The model under review builds one solid part; all positions refer to its coordinate system, in mm. A direction names the side the tool comes from. Round coordinates to 2 decimals unless told otherwise and drop trailing zeros. Answer as CSV lines item,"result". Start each with the question number.
from build123d import *

# Parameters (mm, degrees)
EXTRUDE_1_DEPTH = 15


with BuildPart() as part:
    # 放样1: read off the stored shape, not the designer's step
    # 放样1: loft between two sections, ruled curve by curve
    loft_1_from = [
        Edge.make_bspline([(157.289403045, 194.319437241, 200), (545.928277528, -120.259368848, 200), (231.349471438, -508.898243331, 200), (-157.289403045, -194.319437241, 200), (-545.928277528, 120.259368848, 200), (-231.349471438, 508.898243331, 200), (157.289403045, 194.319437241, 200)], [0, 0, 0, 0, 0.5, 0.5, 0.5, 1, 1, 1, 1], 3, [1, 0.333333333, 0.333333333, 1, 0.333333333, 0.333333333, 1]),
    ]
    loft_1_to = [
        Edge.make_bspline([(42.317097013, 26.631997679, 0), (95.581092372, -58.002196347, 0), (10.946898346, -111.266191705, 0), (-42.317097013, -26.631997679, 0), (-95.581092372, 58.002196347, 0), (-10.946898346, 111.266191705, 0), (42.317097013, 26.631997679, 0)], [0, 0, 0, 0, 0.5, 0.5, 0.5, 1, 1, 1, 1], 3, [1, 0.333333333, 0.333333333, 1, 0.333333333, 0.333333333, 1]),
    ]
    loft_1 = Solid(Shell([*[Face.make_surface_from_curves(loft_1_from[k], loft_1_to[k]) for k in range(1)], Face(Wire(loft_1_from)), Face(Wire(loft_1_to))]))
    add(loft_1)

    # 草图4 → 凸台-拉伸1 (add)
    with BuildSketch(Plane.XY.offset(200)):
        Polygon((0, 250), (-250, 250), (-250, -250), (250, -250), (250, 250), align=None)
    extrude(amount=EXTRUDE_1_DEPTH)


solid = part.part
Item 1: For pin 1 (12 mm diameter, centred on x = 110.5, y = 12, fed in from -Z); pin 2 (8 mm diameter, centred on y = -93.5, z = 191, fed in from +X); pin 3 (4 mm diameter, centred on x = -9.5, z = 127.5, fed in from -Y), all flat-tipped, find the tip position at first contact; note any pin that passes through.
Item 2: Wall thickness on probe 1 along Z at (x, y) = (223.5, -191.5); probe 2 along X at (y, z) = (125, 129.5); probe 3 along Z at (x, y) = (-40.5, -96): over which ranges is each line inside the solid? List them lowest first. Write a range as [from, to].
Item 3: Tool access review of faces 1 (the flat face through (-200, 190, 200)), 2 (the flat face through (189, 200, 200)), 3 (the flat face through (198, -198, 200)), 4 (the flat face through (-200, -189, 200)): name each direction out of +Z, -Z, +X, -X, +Y, -Y from which nothing blocks a thin tool from reaching the whole face with its end or side.
Reported:
1,pin 1,"stops at z = 56.43"
1,pin 2,"stops at x = 226.68"
1,pin 3,"stops at y = -178.4"
2,probe 1,"z = [200, 215]"
2,probe 2,"x = [-127.63, 127.63]"
2,probe 3,"z = [55.47, 215]"
3,face 1,"-Z, -X, +Y"
3,face 2,"-Z, +X, +Y"
3,face 3,"-Z, +X, -Y"
3,face 4,"-Z, -X, -Y"
